Answer from the drawing. Dimensions are ordinates in mm from the lowest x, y and z of the part. A direction names the side the tool comes from. Round coordinates to 2 decimals unless told otherwise and drop trailing zeros. Order: outer loops, then holes, each group sorted by start corner. A loop starts at its lowest first (then second) coordinate and runs counter-clockwise, first axis right, second up. Notation, with made-up numbers: (86, 12) -> (114, 12) arc R11 ccw to (114, 25) -> close; hole circle Ø1 at (42, -13). An arc over 180 degrees is marked (long way). Use a Markdown table: item, result. Add a question column.
1. Section C-C, the plane z = 9 is taken. Give the vertices of the cut face in (x, y), then the cut area to 3 significant figures.
2. Section B-B, the plane y = 3.15 is taken. Give the vertices of the cut face in (x, z), then the cut area to 3 significant figures.
3. Given pin 1 (3 mm diameter, centred on x = 3, z = 8, fed in from -Y); pin 2 (1.6 mm diameter, centred on x = 3, z = 4.5, fed in from +Y), each flat-ended and moving along its own axis, determine where each tip first touches the part or whether it passes through.
4. Consider L1, parallel to Z at x = 3.25, y = 0.5; L2, parallel to X at y = 4.25, z = 6.75; L3, parallel to Y at x = 3, z = 11.25. Determine where each line is inside the solid, lowest interval first. Write a range as [from, to].
5. Section A-A, the plane x = 3.15 is taken. Give the vertices of the cut face in (y, z), then the cut area to 3 significant figures.
6. For the marked faces 1 and 2, determine the directions among +Z, -Z, +X, -X, +Y, -Y from which every point of the face is accessible in a straight line to the end or side of a thin tool.
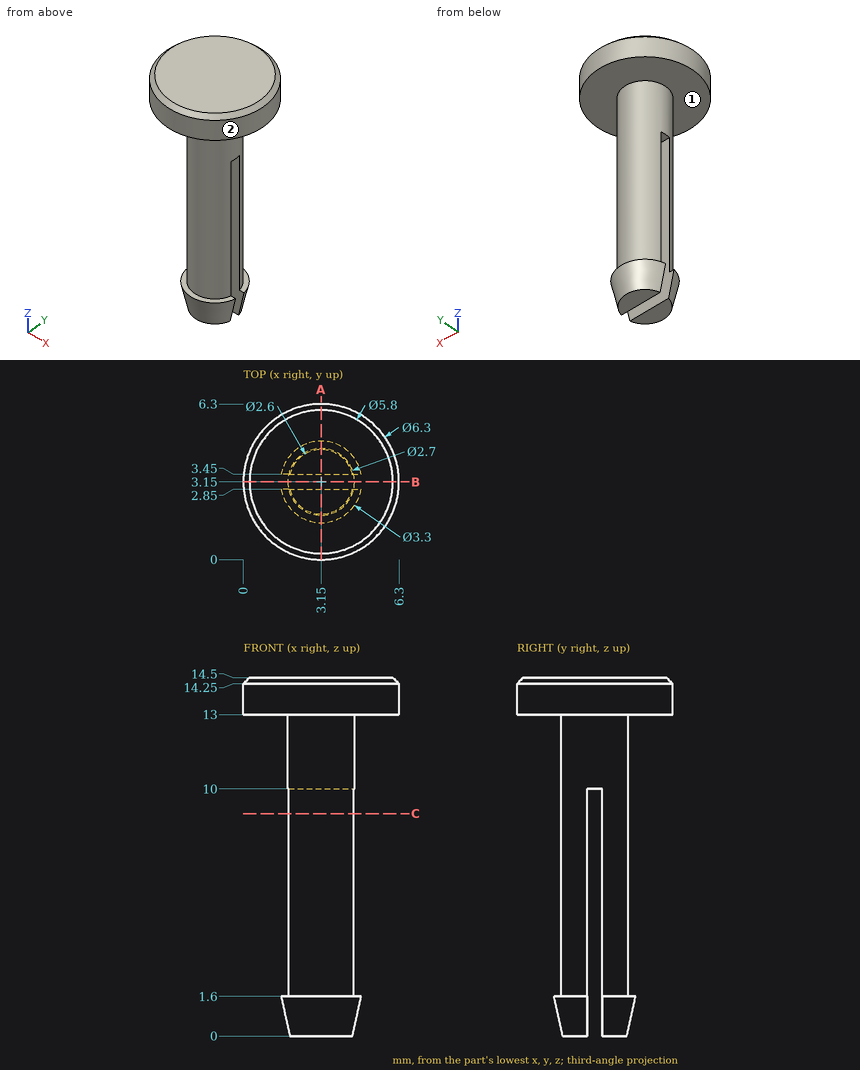
Verdict:
| question | item | result |
|---|---|---|
| 1 | outline | (1.83, 2.85) arc R1.35 ccw to (4.47, 2.85) -> close; (1.83, 3.45) -> (4.47, 3.45) arc R1.35 ccw to start |
| 1 | area | 4.12 mm2 |
| 2 | outline | (0, 13) -> (1.8, 13) -> (1.8, 10) -> (4.5, 10) -> (4.5, 13) -> (6.3, 13) -> (6.3, 14.25) -> (6.05, 14.5) -> (0.25, 14.5) -> (0, 14.25) -> close |
| 2 | area | 17.5 mm2 |
| 3 | pin 1 | stops at y = 1.8 |
| 3 | pin 2 | stops at y = 4.5 |
| 4 | L1 | z = [13, 14.5] |
| 4 | L2 | x = [2.37, 3.93] |
| 4 | L3 | y = [1.81, 4.49] |
| 5 | outline | (0, 13) -> (1.8, 13) -> (1.8, 1.6) -> (1.5, 1.6) -> (1.85, 0) -> (2.85, 0) -> (2.85, 10) -> (3.45, 10) -> (3.45, 0) -> (4.45, 0) -> (4.8, 1.6) -> (4.5, 1.6) -> (4.5, 13) -> (6.3, 13) -> (6.3, 14.25) -> (6.05, 14.5) -> (0.25, 14.5) -> (0, 14.25) -> close |
| 5 | area | 38.9 mm2 |
| 6 | face 1 | none |
| 6 | face 2 | +Z, -Z |
